Can you work these out from the model? Positions are in its coordinate system, mm. A direction names the side the tool comes from. Round coordinates to 2 decimals unless told otherwise and drop trailing zeros. Loops run counter-clockwise (first coordinate to the right, second up) from the corner with the lowest first, then second, coordinate; pieces in that order, holes last. Notation, with made-up numbers: (-13, -14) -> (3, -14) arc R22 ccw to (3, 10) -> close; hole circle Ø6 at (-8.5, 40). An arc over 180 degrees is marked (long way). Answer as a JSON object with one key per item and string values.
```python
from build123d import *

# Parameters (mm, degrees)
SKETCH1_R           = 15
BOSS_EXTRUDE1_DEPTH = 305
SKETCH2_R           = 22.5
BOSS_EXTRUDE2_DEPTH = 8
SKETCH3_R           = 31.5
BOSS_EXTRUDE3_DEPTH = 12.7
SKETCH4_R           = 9.5
BOSS_EXTRUDE5_DEPTH = 7
FILLET1_R           = 2.5


with BuildPart() as part:
    # Sketch1 → Boss-Extrude1 (new body)
    with BuildSketch(Plane(origin=(0, 0, 0), x_dir=(1, 0, 0), z_dir=(0, 1, 0))):
        with Locations(Location((0, 0, 0), (0, 0, 270))):
            Circle(SKETCH1_R)
    extrude(amount=BOSS_EXTRUDE1_DEPTH)

    # Sketch2 → Boss-Extrude2 (add)
    with BuildSketch(Plane(origin=(0, 305, 0), x_dir=(1, 0, 0), z_dir=(0, 1, 0))):
        with Locations(Location((0, 0, 0), (0, 0, 270))):
            Circle(SKETCH2_R)
    extrude(amount=BOSS_EXTRUDE2_DEPTH)

    # Sketch3 → Boss-Extrude3 (add)
    with BuildSketch(Plane.XZ):
        with Locations(Location((0, 0, 0), (0, 0, 270))):
            Circle(SKETCH3_R)
    extrude(amount=BOSS_EXTRUDE3_DEPTH)

    # Sketch4 → Boss-Extrude5 (add, symmetric)
    with BuildSketch(Plane(origin=(0, 0, 0), x_dir=(0, 0, -1), z_dir=(1, 0, 0))):
        with BuildLine():
            Line((-28.5, -12.7), (28.5, -12.7))
            ThreePointArc((28.5, -12.7), (21.470051482, -24.357649102), (18.999946854, -37.744939413))
            ThreePointArc((18.999946854, -37.744939413), (0, -56.7), (-18.999946854, -37.744939413))
            ThreePointArc((-18.999946854, -37.744939413), (-21.470051482, -24.357649102), (-28.5, -12.7))
        make_face()
        with Locations((0, -37.7)):
            Circle(SKETCH4_R, mode=Mode.SUBTRACT)
    extrude(amount=BOSS_EXTRUDE5_DEPTH, both=True)

    # Fillet1
    fillet1_edges = [part.edges().sort_by_distance(p)[0] for p in [
        (0, 0, 31.5),
        (7, -24.357649102, -21.470051482),
        (7, -24.357649102, 21.470051482),
        (7, -56.7, 0),
        (-7, -24.357649102, -21.470051482),
        (-7, -24.357649102, 21.470051482),
        (-7, -56.7, 0),
        (0, 305, -22.5),
        (0, 313, -22.5),
    ]]
    fillet(fillet1_edges, radius=FILLET1_R)


solid = part.part
```
Q1. On a 3-axis mill with a long thin cutter (end or side, diameter ignored), from which of +Z, -Z, +X, -X, +Y, -Y can I reach the whole of each face in a straight line? I mean faces 4 (the flat face through (7, -24, 0)), 5 (the flat face through (-7, -24, 0)), 6 (the cylindrical face through (0.66, 150.365, -14.985)). Say none if no direction works.
Determined:
{"face 4": "+Z, -Z, +X, -Y", "face 5": "+Z, -Z, -X, -Y", "face 6": "none"}
Q2. I want a section at C-C, the plane y = 263.5. Write out the boundary of the cut face in (x, z).
Determined:
{"outline": "circle Ø30 at (0, 0)"}
Q3. I want a section at A-A, the plane x = 0. Write out the boundary of the cut face in (y, z).
Determined:
{"outline": "(-37.74, -19) arc R38 cw to (-12.7, -28.5) -> (-12.7, -31.5) -> (-2.5, -31.5) arc R2.5 ccw to (0, -29) -> (0, -15) -> (305, -15) -> (305, -20) arc R2.5 ccw to (307.5, -22.5) -> (310.5, -22.5) arc R2.5 ccw to (313, -20) -> (313, 20) arc R2.5 ccw to (310.5, 22.5) -> (307.5, 22.5) arc R2.5 ccw to (305, 20) -> (305, 15) -> (0, 15) -> (0, 29) arc R2.5 ccw to (-2.5, 31.5) -> (-12.7, 31.5) -> (-12.7, 28.5) arc R38 cw to (-37.74, 19) arc R19 ccw to start; hole circle Ø19 at (-37.7, 0)"}
Q4. I'm going to push flat-ended pins straight in: pin 1 (5 mm diameter, centred on x = -6.5, z = -2, fed in from -Y); pin 2 (21 mm diameter, centred on y = -35, z = 8.5, fed in from +X); pin 3 (1 mm diameter, centred on y = 246, z = -10, fed in from +X). Where does each tip first touch, or does it pass through?
Determined:
{"pin 1": "y = -56.69", "pin 2": "x = 7", "pin 3": "x = 11.61"}
Q5. We'd pull the mould along Y, two halves only. Please class faces 1 (the flat face through (0, 313, 0)), 2 (the flat face through (7.4, -12.7, 0.4)), 3 (the flat face through (15, 305, 3)): pulls with the +Y half, pulls with the -Y half, needs draft (parallel to the pull), parting line crosses it, or undercut.
Determined:
{"face 1": "pulls with the +Y half", "face 2": "pulls with the -Y half", "face 3": "undercut"}
Q6. If I drill on L1, parallel to Y at x = -1.5, z = 0; L2, parallel to Z at x = -2, y = -37; L3, parallel to Y at x = 15, z = -18.5, over which ranges is the centre line in solid material (lowest first)? Write a range as [from, to].
Determined:
{"L1": "[-56.7, -47.2], [-28.2, 313]", "L2": "[-19.01, -9.47], [9.47, 19.01]", "L3": "[-12.7, 0]"}
Q7. I want a section at B-B, the plane z = 0. Write out the boundary of the cut face in (x, y), then the cut area to 3 significant figures.
Determined:
{"outline": "(-31.5, -12.7) -> (-7, -12.7) -> (-7, -28.2) -> (7, -28.2) -> (7, -12.7) -> (31.5, -12.7) -> (31.5, -2.5) arc R2.5 ccw to (29, 0) -> (15, 0) -> (15, 305) -> (20, 305) arc R2.5 ccw to (22.5, 307.5) -> (22.5, 310.5) arc R2.5 ccw to (20, 313) -> (-20, 313) arc R2.5 ccw to (-22.5, 310.5) -> (-22.5, 307.5) arc R2.5 ccw to (-20, 305) -> (-15, 305) -> (-15, 0) -> (-29, 0) arc R2.5 ccw to (-31.5, -2.5) -> close; (-7, -54.2) arc R2.5 ccw to (-4.5, -56.7) -> (4.5, -56.7) arc R2.5 ccw to (7, -54.2) -> (7, -47.2) -> (-7, -47.2) -> close", "area": "10,600 mm²"}
